The listing builds one solid part. Answer for the finished solid, in the listing's coordinates (mm). Face numbers are marked on the shaded views. Round coordinates to 2 decimals unless told otherwise and drop trailing zeros. Return JSON: item names as keys, results as strings. Group by question number.
(1) Section A-A, the plane y = 6 is taken. Give the number of separate pieces and of enclosed holes in the cut face, then the cut area to 3 significant figures.
(2) Each of these flat-tipped pins is pushed along its axis until it touches: pin 1 (5 mm diameter, centred on y = 19, z = -11, fed in from +X); pin 2 (6 mm diameter, centred on x = 1.5, z = -19.5, fed in from -Y); pin 3 (5 mm diameter, centred on x = 2, y = 14.5, fed in from -Z); pin 4 (8 mm diameter, centred on x = -3, z = -21, fed in from +Y). Where does it stop, or does it pass through?
(3) Determine the mould class of the marked faces 1, 2 and 3 for opening direction Z: +Z half, -Z half, draft (parallel to the pull), parting line (faces both ways), or undercut.
(4) Find the intervals of material crossed by line 1 along X through (y, z) = (5, 0); line 2 along Y through (x, z) = (-0.75, -20.5); line 3 along Z through (x, y) = (1, 1.5), in increasing order. Write a range as [from, to].
```python
from build123d import *

# Parameters (mm, degrees)
SKETCH1_R                = 8.5
BOSS_EXTRUDE1_DEPTH      = 25
BOSS_EXTRUDE2_REACH      = 44.799
BOSS_EXTRUDE2_END_RADIUS = 8.5
SKETCH4_R                = 5.5
SHELL1_START             = -23.159597133
SHELL1_2_OUTLINE_R       = 2
SHELL1_2_DEPTH           = 26.159597133


with BuildPart() as part:
    # Sketch1 → Boss-Extrude1 (new body)
    with BuildSketch(Plane(origin=(0, 0, 0), x_dir=(1, 0, 0), z_dir=(0, 1, 0))):
        with Locations(Location((0, 0, 0), (0, 0, 270))):
            Circle(SKETCH1_R)
    extrude(amount=BOSS_EXTRUDE1_DEPTH)

    # Sketch2 → Revolve1 (revolve)
    with BuildSketch(Plane(origin=(0, 0, 0), x_dir=(0, 0, -1), z_dir=(1, 0, 0))):
        with BuildLine():
            Line((0, 25), (0, 30))
            ThreePointArc((0, 30), (5.112034816, 28.965459187), (8.5, 25))
            Line((8.5, 25), (0, 25))
        make_face()
    revolve(axis=Axis((0, 25, 0), (0, 1, 0)))

    # Boss-Extrude2: up to this cylinder (the profile starts outside it)
    boss_extrude2_end = Plane(origin=(0, 9.739396, 0), z_dir=(0, -1, 0)) * Cylinder(BOSS_EXTRUDE2_END_RADIUS, 107.598, mode=Mode.PRIVATE)
    # Sketch4 → Boss-Extrude2 (add, up to the surface)
    with BuildSketch(Plane(origin=(0, 9.7393957, -28.190778624), x_dir=(-1, 0, 0), z_dir=(0, -0.3420201433256657, -0.9396926207859096)), mode=Mode.PRIVATE) as boss_extrude2_sk1:
        with Locations(Location((0, 0, 0), (0, 0, 90))):
            Circle(SKETCH4_R)
    boss_extrude2_tool1 = extrude(boss_extrude2_sk1.sketch, amount=-BOSS_EXTRUDE2_REACH, mode=Mode.PRIVATE) - boss_extrude2_end
    add(boss_extrude2_tool1.solids().sort_by_distance((0, 9.739396, -28.190779))[0])

    # Shell1: read off the stored shape, not the designer's step
    # Shell1 outline → Shell1 (revolve, cut)
    with BuildSketch(Plane.XY):
        with BuildLine():
            Line((0, 26.444357479), (0, 0))
            Line((0, 0), (5, 0))
            Line((5, 0), (5, 24.236519229))
            add(Edge.make_bspline(
                [(5, 24.236519229), (4.572818275, 25.014193993), (3.910724446, 25.762107964), (3.017623345, 26.318986428), (2.002643397, 26.569985468), (0.836195706, 26.569985465), (0.619342604, 26.556580246), (0.406891162, 26.530460172), (0.200126847, 26.492663543), (0, 26.444357479)],
                knots=[4.721376583, 4.721376583, 4.721376583, 4.721376583, 4.721376583, 4.721376583, 5.780874766, 5.780874766, 5.780874766, 5.780874766, 6.026709165, 6.026709165, 6.026709165, 6.026709165, 6.026709165, 6.026709165], degree=5, weights=[1, 1, 0.993014221, 0.992005425, 1, 1, 0.999993273, 0.999995808, 1, 1]))
        make_face()
    revolve(axis=Axis((0, 0, 0), (0, 1, 0)), mode=Mode.SUBTRACT)

    # Shell1 2 outline → Shell1 2 (cut)
    with BuildSketch(Plane(origin=(0, 0, 0), x_dir=(1, 0, 0), z_dir=(0, 0.34202014332566616, 0.9396926207859094)).offset(SHELL1_START)):
        with Locations((0, 18.793852416)):
            Circle(SHELL1_2_OUTLINE_R)
    extrude(amount=SHELL1_2_DEPTH, mode=Mode.SUBTRACT)


solid = part.part
```
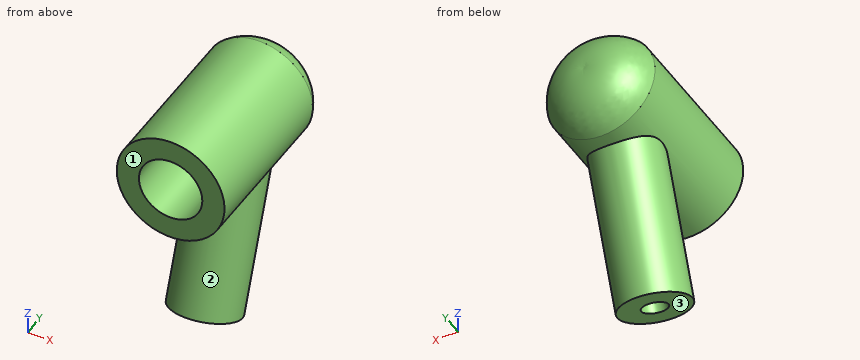
Working result:
{
 "1": {"separate pieces": "2", "enclosed holes": "1", "area": "172 mm^2"},
 "2": {"pin 1": "stops at x = 5.49", "pin 2": "stops at y = 6.04", "pin 3": "stops at z = -30.07", "pin 4": "stops at y = 19.37"},
 "3": {"face 1": "draft", "face 2": "undercut", "face 3": "-Z half"},
 "4": {"line 1": "x = [-8.5, -5], [5, 8.5]", "line 2": "y = [6.74, 10.57], [14.51, 18.34]", "line 3": "z = [-8.44, -4.9], [4.9, 8.44]"}
}
